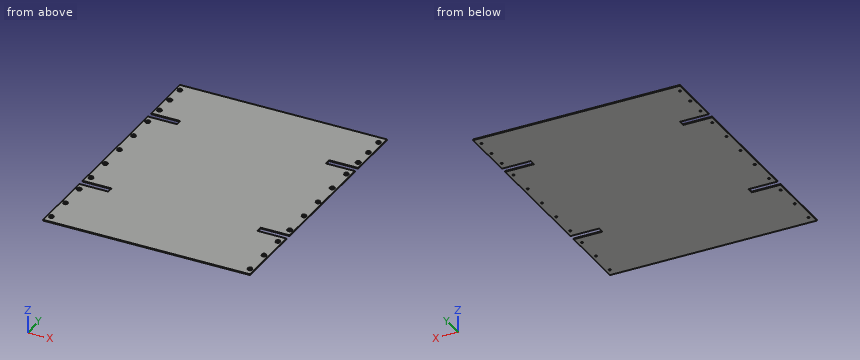
```python
from build123d import *

# Parameters (mm, degrees)
F0_R     = 3.175
F1_DEPTH = 2.54
F2_R     = 6.985
F2_R_2   = 3.175
F3_DEPTH = 2.54


with BuildPart() as f1:
    # F0 (on Top) → F1 (new body)
    with BuildSketch(Plane.XY):
        Polygon((-317.5, -406.4), (317.5, -406.4), (317.5, -190.5), (228.6, -190.5), (228.6, -171.45), (317.5, -171.45), (317.5, 215.9), (228.6, 215.9), (228.6, 234.95), (317.5, 234.95), (317.5, 406.4), (-317.5, 406.4), (-317.5, 234.95), (-228.6, 234.95), (-228.6, 215.9), (-317.5, 215.9), (-317.5, -171.45), (-228.6, -171.45), (-228.6, -190.5), (-317.5, -190.5), align=None)
        with Locations((-304.8, -381)):
            Circle(F0_R, mode=Mode.SUBTRACT)
        with Locations((-304.8, -298.45)):
            Circle(F0_R, mode=Mode.SUBTRACT)
        with Locations((-304.8, -215.9)):
            Circle(F0_R, mode=Mode.SUBTRACT)
        with Locations((-304.8, -146.05)):
            Circle(F0_R, mode=Mode.SUBTRACT)
        with Locations((-304.8, -61.9125)):
            Circle(F0_R, mode=Mode.SUBTRACT)
        with Locations((304.8, -381)):
            Circle(F0_R, mode=Mode.SUBTRACT)
        with Locations((304.8, -298.45)):
            Circle(F0_R, mode=Mode.SUBTRACT)
        with Locations((304.8, -215.9)):
            Circle(F0_R, mode=Mode.SUBTRACT)
        with Locations((304.8, -146.05)):
            Circle(F0_R, mode=Mode.SUBTRACT)
        with Locations((304.8, -61.9125)):
            Circle(F0_R, mode=Mode.SUBTRACT)
        with Locations((-304.8, 22.225)):
            Circle(F0_R, mode=Mode.SUBTRACT)
        with Locations((-304.8, 106.3625)):
            Circle(F0_R, mode=Mode.SUBTRACT)
        with Locations((-304.8, 190.5)):
            Circle(F0_R, mode=Mode.SUBTRACT)
        with Locations((-304.8, 260.35)):
            Circle(F0_R, mode=Mode.SUBTRACT)
        with Locations((-304.8, 320.675)):
            Circle(F0_R, mode=Mode.SUBTRACT)
        with Locations((-304.8, 381)):
            Circle(F0_R, mode=Mode.SUBTRACT)
        with Locations((304.8, 22.225)):
            Circle(F0_R, mode=Mode.SUBTRACT)
        with Locations((304.8, 106.3625)):
            Circle(F0_R, mode=Mode.SUBTRACT)
        with Locations((304.8, 190.5)):
            Circle(F0_R, mode=Mode.SUBTRACT)
        with Locations((304.8, 260.35)):
            Circle(F0_R, mode=Mode.SUBTRACT)
        with Locations((304.8, 320.675)):
            Circle(F0_R, mode=Mode.SUBTRACT)
        with Locations((304.8, 381)):
            Circle(F0_R, mode=Mode.SUBTRACT)
    extrude(amount=F1_DEPTH)

    # F2 (on face) → F3 (join)
    with BuildSketch(Plane.XY.offset(2.54)):
        with Locations((304.8, -381)):
            Circle(F2_R)
        with Locations((304.8, -381)):
            Circle(F2_R_2, mode=Mode.SUBTRACT)
        with Locations((304.8, -298.45)):
            Circle(F2_R)
        with Locations((304.8, -298.45)):
            Circle(F2_R_2, mode=Mode.SUBTRACT)
        with Locations((304.8, -215.9)):
            Circle(F2_R)
        with Locations((304.8, -215.9)):
            Circle(F2_R_2, mode=Mode.SUBTRACT)
        with Locations((304.8, -146.05)):
            Circle(F2_R)
        with Locations((304.8, -146.05)):
            Circle(F2_R_2, mode=Mode.SUBTRACT)
        with Locations((304.8, -61.9125)):
            Circle(F2_R)
        with Locations((304.8, -61.9125)):
            Circle(F2_R_2, mode=Mode.SUBTRACT)
        with Locations((304.8, 22.225)):
            Circle(F2_R)
        with Locations((304.8, 22.225)):
            Circle(F2_R_2, mode=Mode.SUBTRACT)
        with Locations((304.8, 106.3625)):
            Circle(F2_R)
        with Locations((304.8, 106.3625)):
            Circle(F2_R_2, mode=Mode.SUBTRACT)
        with Locations((304.8, 190.5)):
            Circle(F2_R)
        with Locations((304.8, 190.5)):
            Circle(F2_R_2, mode=Mode.SUBTRACT)
        with Locations((304.8, 260.35)):
            Circle(F2_R)
        with Locations((304.8, 260.35)):
            Circle(F2_R_2, mode=Mode.SUBTRACT)
        with Locations((304.8, 320.675)):
            Circle(F2_R)
        with Locations((304.8, 320.675)):
            Circle(F2_R_2, mode=Mode.SUBTRACT)
        with Locations((304.8, 381)):
            Circle(F2_R)
        with Locations((304.8, 381)):
            Circle(F2_R_2, mode=Mode.SUBTRACT)
        with Locations((-304.8, 381)):
            Circle(F2_R)
        with Locations((-304.8, 381)):
            Circle(F2_R_2, mode=Mode.SUBTRACT)
        with Locations((-304.8, 320.675)):
            Circle(F2_R)
        with Locations((-304.8, 320.675)):
            Circle(F2_R_2, mode=Mode.SUBTRACT)
        with Locations((-304.8, 260.35)):
            Circle(F2_R)
        with Locations((-304.8, 260.35)):
            Circle(F2_R_2, mode=Mode.SUBTRACT)
        with Locations((-304.8, 190.5)):
            Circle(F2_R)
        with Locations((-304.8, 190.5)):
            Circle(F2_R_2, mode=Mode.SUBTRACT)
        with Locations((-304.8, 106.3625)):
            Circle(F2_R)
        with Locations((-304.8, 106.3625)):
            Circle(F2_R_2, mode=Mode.SUBTRACT)
        with Locations((-304.8, 22.225)):
            Circle(F2_R)
        with Locations((-304.8, 22.225)):
            Circle(F2_R_2, mode=Mode.SUBTRACT)
        with Locations((-304.8, -61.9125)):
            Circle(F2_R)
        with Locations((-304.8, -61.9125)):
            Circle(F2_R_2, mode=Mode.SUBTRACT)
        with Locations((-304.8, -146.05)):
            Circle(F2_R)
        with Locations((-304.8, -146.05)):
            Circle(F2_R_2, mode=Mode.SUBTRACT)
        with Locations((-304.8, -215.9)):
            Circle(F2_R)
        with Locations((-304.8, -215.9)):
            Circle(F2_R_2, mode=Mode.SUBTRACT)
        with Locations((-304.8, -298.45)):
            Circle(F2_R)
        with Locations((-304.8, -298.45)):
            Circle(F2_R_2, mode=Mode.SUBTRACT)
        with Locations((-304.8, -381)):
            Circle(F2_R)
        with Locations((-304.8, -381)):
            Circle(F2_R_2, mode=Mode.SUBTRACT)
    extrude(amount=F3_DEPTH)


solid = f1.part
```
Here's how the part is built. I have some questions about the finished solid (model axes, mm). Coordinates: 2 decimals unless noted, no trailing zeros. Order: outer loops, then holes, each group sorted by start corner. A loop starts at its lowest first (then second) coordinate and runs counter-clockwise, first axis right, second up. Notation, with made-up numbers: M -5,30 L 9,30 A16 cw 9,38 Z; hole C 81.25,17.25 d9. An arc over 180 degrees is marked long. Answer as a JSON object with one key per item and string values. Group by question number.
(1) Suppose I cut it at C-C, the plane x = 192.5. Please give me the cut outline in (y, z).
(2) Suppose I cut it at A-A, the plane z = 3.7. State how many separate pieces and enclosed holes the cut face has, then the cut area to 3 significant figures.
(3) For pin 1 (0.8 mm diameter, centred on y = -180, z = 1.5, fed in from +X); pin 2 (3 mm diameter, centred on y = 228, z = 1, fed in from -X); pin 3 (4 mm diameter, centred on x = -161.5, y = 128.5, fed in from +Z), each with a flat end and sliding along its axis, tell me the tip position at first contact or that it passes through.
(4) Suppose I cut it at B-B, the plane y = -2. Please give me the cut outline in (x, z).
(5) I need wall thicknesses on probe 1 along Y at (x, z) = (256, 1.8); probe 2 along X at (y, z) = (-298.45, 2.4) (3 decimals); probe 3 along X at (y, z) = (381, 2.95) (3 decimals). Which ranges of each line are inside material? Lowest first, please.
Values found:
{
 "1": {"outline": "M -406.4,0 L 406.4,0 L 406.4,2.54 L -406.4,2.54 Z"},
 "2": {"separate pieces": "22", "enclosed holes": "22", "area": "2,680 mm^2"},
 "3": {"pin 1": "stops at x = 228.6", "pin 2": "stops at x = -228.6", "pin 3": "stops at z = 2.54"},
 "4": {"outline": "M -317.5,0 L 317.5,0 L 317.5,2.54 L -317.5,2.54 Z"},
 "5": {"probe 1": "y = -406.4 to -190.5, -171.45 to 215.9, 234.95 to 406.4", "probe 2": "x = -317.5 to -307.975, -301.625 to 301.625, 307.975 to 317.5", "probe 3": "x = -311.785 to -307.975, -301.625 to -297.815, 297.815 to 301.625, 307.975 to 311.785"}
}
